Work out the finished part from the listing and answer in its coordinate system (mm). A direction names the side the tool comes from. Round coordinates to 2 decimals unless told otherwise and drop trailing zeros. Write each loop counter-clockwise with the first axis right and the second up, starting at its lowest first coordinate (ties: lowest second). Pieces come first, ordered by that corner, then holes. Notation, with made-up numbers: M 88.5,76.5 L 115.5,76.5 A28 cw 115.5,104.5 Z; hole C 28.5,51.25 d10. An arc over 180 degrees is marked long. Answer in a Markdown table with one row per item.
```python
from build123d import *

# Parameters (mm, degrees)
SKETCH1_W           = 2
SKETCH1_H           = 2
BOSS_EXTRUDE1_DEPTH = 2.8
SKETCH2_W           = 5
SKETCH2_H           = 5
BOSS_EXTRUDE2_DEPTH = 0.2
SKETCH3_R           = 0.5
BOSS_EXTRUDE3_DEPTH = 1
SCALE1_SCALE        = 6


with BuildPart() as part:
    # Sketch1 → Boss-Extrude1 (new body)
    with BuildSketch(Plane(origin=(0, 0, 0), x_dir=(1, 0, 0), z_dir=(0, 1, 0))):
        Rectangle(SKETCH1_W, SKETCH1_H)
    extrude(amount=BOSS_EXTRUDE1_DEPTH)

    # Sketch2 → Boss-Extrude2 (add)
    with BuildSketch(Plane(origin=(0, 0, 0), x_dir=(1, 0, 0), z_dir=(0, 1, 0))):
        Rectangle(SKETCH2_W, SKETCH2_H)
    extrude(amount=-BOSS_EXTRUDE2_DEPTH)

    # Sketch3 → Boss-Extrude3 (add)
    with BuildSketch(Plane(origin=(0, -0.2, 0), x_dir=(-1, 0, 0), z_dir=(0, -1, 0))):
        with Locations(Location((0, 0, 0), (0, 0, 90))):
            Circle(SKETCH3_R)
    extrude(amount=BOSS_EXTRUDE3_DEPTH)


with BuildPart() as part_1:
    # Scale1: scaled about (0, 0.861341085, 0)
    add(part.part.scale(SCALE1_SCALE).moved(Location((0, -4.306705425, 0))))


solid = part_1.part
```
1. Consider line 1 along Y through (x, z) = (-0.25, 13.25); line 2 along X through (y, z) = (7.75, -4.5); line 3 along Y through (x, z) = (-5, 4.5). Determine where each line is inside the solid, lowest interval first. Write a range as from..to.
Calculated:
| item | result |
|---|---|
| line 1 | y = -5.51..-4.31 |
| line 2 | x = -6..6 |
| line 3 | y = -5.51..12.49 |
2. The part is cut by section A-A (z = 0). Determine the outline of the cut face in (x, y).
Calculated:
| item | result |
|---|---|
| outline | M -15,-5.51 L -3,-5.51 L -3,-11.51 L 3,-11.51 L 3,-5.51 L 15,-5.51 L 15,-4.31 L 6,-4.31 L 6,12.49 L -6,12.49 L -6,-4.31 L -15,-4.31 Z |
3. The part is cut by section B-B (x = 0). Determine the outline of the cut face in (y, z).
Calculated:
| item | result |
|---|---|
| outline | M -11.51,-3 L -5.51,-3 L -5.51,-15 L -4.31,-15 L -4.31,-6 L 12.49,-6 L 12.49,6 L -4.31,6 L -4.31,15 L -5.51,15 L -5.51,3 L -11.51,3 Z |
4. The part is cut by section C-C (y = -2.25). Determine the outline of the cut face in (x, z).
Calculated:
| item | result |
|---|---|
| outline | M -6,-6 L 6,-6 L 6,6 L -6,6 Z |
5. A tool of negligible diameter and unlimited length cuts with its end or side. For faces 1 (the cylindrical face through (0.9, -8.46, -2.86)), 2 (the flat face through (0, 4, -6)), 3 (the flat face through (0, 4, 6)), 4 (the flat face through (6, 4, 0)), 5 (the flat face through (-6, 4, 0)), from which of +Z, -Z, +X, -X, +Y, -Y can it reach the whole face along a straight path? Write none if from no direction.
Calculated:
| item | result |
|---|---|
| face 1 | -Y |
| face 2 | -Z, +X, -X, +Y |
| face 3 | +Z, +X, -X, +Y |
| face 4 | +Z, -Z, +X, +Y |
| face 5 | +Z, -Z, -X, +Y |
6. The part is cut by section D-D (x = -4.5). Determine the outline of the cut face in (y, z), plus the area to 3 significant figures.
Calculated:
| item | result |
|---|---|
| outline | M -5.51,-15 L -4.31,-15 L -4.31,-6 L 12.49,-6 L 12.49,6 L -4.31,6 L -4.31,15 L -5.51,15 Z |
| area | 238 mm² |
7. Given pin 1 (6 mm diameter, centred on x = 0.5, y = 7.5, fed in from +Z); pin 2 (5 mm diameter, centred on x = -3.5, y = -0.5, fed in from -Z); pin 3 (5 mm diameter, centred on x = -10.5, z = -7, fed in from +Y); pin 4 (15 mm diameter, centred on x = 4, z = -7.5, fed in from +Y), each flat-ended and moving along its own axis, determine where each tip first touches the part or whether it passes through.
Calculated:
| item | result |
|---|---|
| pin 1 | stops at z = 6 |
| pin 2 | stops at z = -6 |
| pin 3 | stops at y = -4.31 |
| pin 4 | stops at y = 12.49 |
